The listing builds one solid part. Answer for the finished solid, in the listing's coordinates (mm). Face numbers are marked on the shaded views. A direction names the side the tool comes from. Coordinates: 2 decimals unless noted, no trailing zeros. Write each loop counter-clockwise with the first axis right and the second up, starting at its lowest first coordinate (ties: lowest second). Pieces come first, ordered by that corner, then holes.
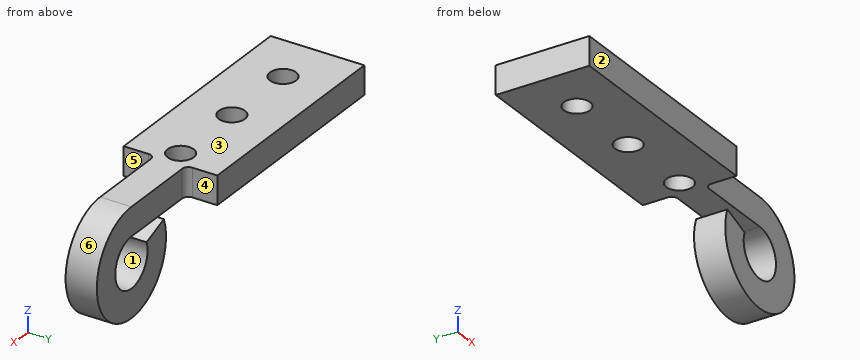
from build123d import *

# Parameters (mm, degrees)
BASE_FLANGE1_DEPTH      = 15
CUT_EXTRUDE1_DEPTH      = 14
CUT_EXTRUDE1_DEPTH_BACK = 10
SKETCH6_W               = 22.14
SKETCH6_H               = 5
SKETCH7_R               = 2.1
CUT_EXTRUDE2_DEPTH      = 10
FILLET2_R               = 1


# Sheet-metal steps are written as plain solids
with BuildPart() as part:
    # Sketch1 → Base-Flange1 (new body)
    with BuildSketch(Plane(origin=(0, 0, 0), x_dir=(1, 0, 0), z_dir=(0, 1, 0))):
        with BuildLine():
            Line((0, 0), (50, 0))
            ThreePointArc((50, 0), (52.294305745, 7.276608177), (46.241229517, 2.631919427))
            Line((46.241229517, 2.631919427), (41.94683424, 1.068887372))
            ThreePointArc((41.94683424, 1.068887372), (54.91555006, 11.02013302), (50, -4.57))
            Line((50, -4.57), (0, -4.57))
            Line((0, -4.57), (0, 0))
        make_face()
    extrude(amount=BASE_FLANGE1_DEPTH)

    # Sketch6 → Cut-Extrude1 (cut, two sides: drawn at the far end of the back side and taken through both)
    with BuildSketch(Plane(origin=(0, 0, 0), x_dir=(-1, 0, 0), z_dir=(0, 0, -1)).offset(-CUT_EXTRUDE1_DEPTH_BACK)):
        with Locations((-47.5, 12.5)):
            Rectangle(SKETCH6_W, SKETCH6_H)
        with Locations((-47.5, 2.5)):
            Rectangle(SKETCH6_W, SKETCH6_H)
    extrude(amount=CUT_EXTRUDE1_DEPTH + CUT_EXTRUDE1_DEPTH_BACK, mode=Mode.SUBTRACT)

    # Sketch7 → Cut-Extrude2 (cut)
    with BuildSketch(Plane(origin=(0, 0, 0), x_dir=(-1, 0, 0), z_dir=(0, 0, -1))):
        with Locations((-21.23, 7.5)):
            Circle(SKETCH7_R)
        with Locations((-33.93, 7.5)):
            Circle(SKETCH7_R)
        with Locations((-8.53, 7.5)):
            Circle(SKETCH7_R)
    extrude(amount=-CUT_EXTRUDE2_DEPTH, mode=Mode.SUBTRACT)

    # Fillet2
    fillet2_edges = [part.edges().sort_by_distance(p)[0] for p in [
        (36.43, 10, 2.285),
        (36.43, 5, 2.285),
    ]]
    fillet(fillet2_edges, radius=FILLET2_R)


solid = part.part
Q1. The part is cut by section D-D, the plane x = 11.5. Write down the section's boundary in (y, z).
Answers below:
outline: (0, 0) - (15, 0) - (15, 4.57) - (0, 4.57) - close
Q2. Given pin 1 (9 mm diameter, centred on x = 50, z = -4, fed in from +Y); pin 2 (1.2 mm diameter, centred on y = 3, z = 2, fed in from +X); pin 3 (8.5 mm diameter, centred on x = 44, z = -6.5, fed in from -Y); pin 4 (3.5 mm diameter, centred on x = 33.93, y = 7.5, fed in from +Z), each flat-ended and moving along its own axis, determine where each tip first touches the part or whether it passes through.
Answers below:
pin 1: stops at y = 10
pin 2: stops at x = 36.43
pin 3: stops at y = 5
pin 4: passes through
Q3. Which of the six approach directions +Z, -Z, +X, -X, +Y, -Y give full straight-line access (tool end or side, diameter ignored) to the marked faces 4, 5 and 6?
Answers below:
face 4: +Z, -Z, +X, +Y
face 5: +Z, -Z, +X, -Y
face 6: +Y, -Y
Q4. Find the intervals of material crossed by probe 1 along Z at (x, y) = (50, 8.5); probe 2 along X at (y, z) = (6.8, -4); probe 3 along Y at (x, z) = (33.93, 1.75), in increasing order.
Answers below:
probe 1: z = -12.57 to -8, 0 to 4.57
probe 2: x = 41.43 to 46, 54 to 58.57
probe 3: y = 0 to 5.4, 9.6 to 15
Q5. The part is cut by section B-B, the plane z = -4. Write down the section's boundary in (x, y).
Answers below:
outline: (41.43, 5) - (46, 5) - (46, 10) - (41.43, 10) - close; (54, 5) - (58.57, 5) - (58.57, 10) - (54, 10) - close
Q6. The part is cut by section C-C, the plane y = 7.5. Write down the section's boundary in (x, z), then the cut area to 3 significant figures.
Answers below:
outline: (0, 0) - (6.43, 0) - (6.43, 4.57) - (0, 4.57) - close; (10.63, 0) - (19.13, 0) - (19.13, 4.57) - (10.63, 4.57) - close; (23.33, 0) - (31.83, 0) - (31.83, 4.57) - (23.33, 4.57) - close; (36.03, 0) - (50, 0) arc R4 cw (long way) to (46.24, -2.63) - (41.95, -1.07) arc R8.57 ccw (long way) to (50, 4.57) - (36.03, 4.57) - close
area: 316 mm2
Q7. Determine the mould class of the marked faces 1, 2 and 3 for opening direction Z: released by +Z, released by -Z, zero draft, split by the parting line, or undercut.
Answers below:
face 1: undercut
face 2: zero draft
face 3: released by +Z
Q8. The part is cut by section A-A, the plane x = 33.93. Write down the section's boundary in (y, z).
Answers below:
outline: (0, 0) - (5.4, 0) - (5.4, 4.57) - (0, 4.57) - close; (9.6, 0) - (15, 0) - (15, 4.57) - (9.6, 4.57) - close
